The drawing under review shows one solid part. Ordinate dimensions are in mm from its lowest x, y, z. A direction names the side the tool comes from. Give positions to 0.01 mm unless a question says otherwise; leave off trailing zeros. Loops run counter-clockwise (first coordinate to the right, second up) from the corner with the lowest first, then second, coordinate; pieces in that order, holes last. Notation, with made-up numbers: (-17.75, -28.75) - (-6.75, -28.75) arc R19 ccw to (-6.75, -17.75) - close; hole circle Ø9 at (56, 13). An arc over 180 degrees is marked (long way). Return JSON: item names as keys, results as strings. Group by question number.
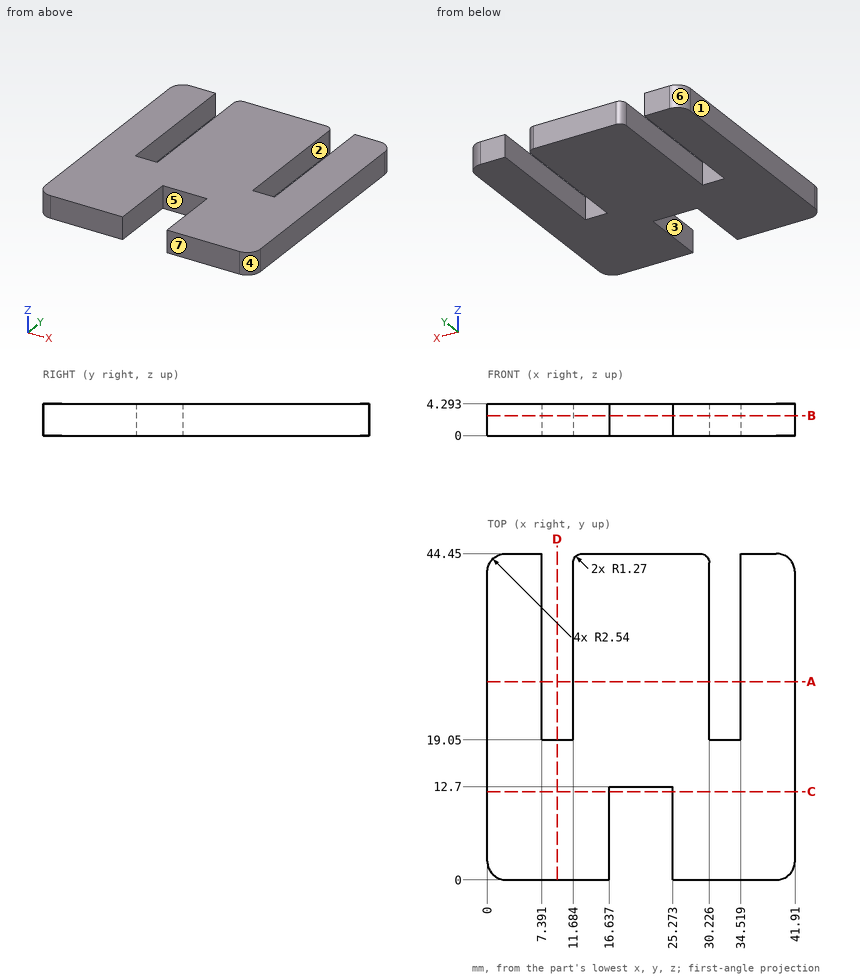
1) We need section A-A, the plane y = 27. Write out the cut boundary in (x, z), plus the area to 3 significant figures.
2) Draft analysis for pull direction X (two halves, no side actions). For the marked faces 4, 5, 6 and 7, state which applies: +X half, -X half, draft (parallel to the pull), parting line (faces both ways), or undercut.
3) We need section C-C, the plane y = 12. Write out the cut boundary in (x, z).
4) Tool access review of the marked faces 1, 2 and 3: name each direction out of +Z, -Z, +X, -X, +Y, -Y from which nothing blocks a thin tool from reaching the whole face with its end or side.
5) We need section D-D, the plane x = 9.5. Write out the cut boundary in (y, z).
6) To check wall thickness, follow line 1 (X direction, y = 25, z = 1.2); line 2 (X direction, y = 11.5, z = 0.4); line 3 (Y direction, x = 19.5, z = 2.8). State the ranges of each line that lie inside material, in increasing order.
7) For pin 1 Ø8 at (x, y) = (37.5, 23) entering from -Z; pin 2 Ø2 at (x, z) = (9.5, 1.5) entering from +Y, all flat-tipped, find the tip position at first contact; note any pin that passes through.
8) We need section B-B, the plane z = 2.7. Write out the cut boundary in (x, y), plus the area to 3 significant figures.
Findings:
{
 "1": {"outline": "(0, 0) - (7.39, 0) - (7.39, 4.29) - (0, 4.29) - close; (11.68, 0) - (30.23, 0) - (30.23, 4.29) - (11.68, 4.29) - close; (34.52, 0) - (41.91, 0) - (41.91, 4.29) - (34.52, 4.29) - close", "area": "143 mm^2"},
 "2": {"face 4": "+X half", "face 5": "undercut", "face 6": "-X half", "face 7": "draft"},
 "3": {"outline": "(0, 0) - (16.64, 0) - (16.64, 4.29) - (0, 4.29) - close; (25.27, 0) - (41.91, 0) - (41.91, 4.29) - (25.27, 4.29) - close"},
 "4": {"face 1": "+Z, -Z, -X, +Y, -Y", "face 2": "+Z, -Z, +Y", "face 3": "+Z, -Z, -Y"},
 "5": {"outline": "(0, 0) - (19.05, 0) - (19.05, 4.29) - (0, 4.29) - close"},
 "6": {"line 1": "x = 0 to 7.39, 11.68 to 30.23, 34.52 to 41.91", "line 2": "x = 0 to 16.64, 25.27 to 41.91", "line 3": "y = 12.7 to 44.45"},
 "7": {"pin 1": "stops at z = 0", "pin 2": "stops at y = 19.05"},
 "8": {"outline": "(0, 2.54) arc R2.54 ccw to (2.54, 0) - (16.64, 0) - (16.64, 12.7) - (25.27, 12.7) - (25.27, 0) - (39.37, 0) arc R2.54 ccw to (41.91, 2.54) - (41.91, 41.91) arc R2.54 ccw to (39.37, 44.45) - (34.52, 44.45) - (34.52, 19.05) - (30.23, 19.05) - (30.23, 43.18) arc R1.27 ccw to (28.96, 44.45) - (12.95, 44.45) arc R1.27 ccw to (11.68, 43.18) - (11.68, 19.05) - (7.39, 19.05) - (7.39, 44.45) - (2.54, 44.45) arc R2.54 ccw to (0, 41.91) - close", "area": "1,530 mm^2"}
}
